Geometry: final body of the model. Coordinates: model frame, mm. A direction names the side the tool comes from. Coordinates: 2 decimals unless noted, no trailing zeros. Loops run counter-clockwise (first coordinate to the right, second up) from the corner with the lowest first, then second, coordinate; pieces in that order, holes last. Notation, with made-up numbers: (-12.5, -22.75) - (29.5, -22.75) arc R28 cw to (29.5, 15.25) - close; hole circle Ø2 at (12.25, 51.25). An arc over 180 degrees is marked (long way). Return JSON: item names as keys, results as strings.
Autodesk Inventor part; units mm, degrees
ref_plane "YZ Plane" through (0, 0, 0) normal (1, 0, 0) x (0, 1, 0)
ref_plane "XZ Plane" through (0, 0, 0) normal (0, 1, 0) x (-1, 0, 0)
ref_plane "XY Plane" through (0, 0, 0) normal (0, 0, 1) x (1, 0, 0)
sketch "Sketch1" plane through (0, 0, 0) normal (0, 0, 1) x (1, 0, 0)
  line L0 (393.6245, -95.4118) -> (-70.3755, -95.4118)
  line L1 (-70.3755, 4.5882) -> (17.6245, 4.5882)
  line L2 (117.6245, 4.5882) -> (205.6245, 4.5882)
  line L3 (305.6245, 4.5882) -> (393.6245, 4.5882)
  line L4 (-88.3755, -15.4118) -> (-70.3755, -15.4118)
  line L5 (-70.3755, -75.4118) -> (-88.3755, -75.4118)
  line L6 (-88.3755, -75.4118) -> (-88.3755, -15.4118)
  line L7 (-70.3755, -95.4118) -> (-70.3755, -75.4118)
  line L8 (-70.3755, -15.4118) -> (-70.3755, 4.5882)
  line L9 (393.6245, -15.4118) -> (411.6245, -15.4118)
  line L10 (411.6245, -15.4118) -> (411.6245, -75.4118)
  line L11 (411.6245, -75.4118) -> (393.6245, -75.4118)
  line L12 (393.6245, 4.5882) -> (393.6245, -15.4118)
  line L13 (393.6245, -75.4118) -> (393.6245, -95.4118)
  line L14 (17.6245, 4.5882) -> (117.6245, 4.5882)
  line L15 (205.6245, 4.5882) -> (305.6245, 4.5882)
  point P0 (0, 0)
  dimension "d0" = 464
  dimension "d4" = 100
  dimension "d9" = 100
  dimension "d13" = 18
  dimension "d14" = 60
  dimension "d17" = 20
  dimension "d19" = 60
  dimension "d20" = 18
  dimension "d21" = 100
extrude "Extrusion1" add sketch "Sketch1" along normal blind 18
sketch "Sketch3" plane through (0, 0, 18) normal (0, 0, 1) x (1, 0, 0)
  line L0 (-70.3755, -15.4118) -> (-71.5069, -14.2805)
  line L1 (-70.3755, -15.4118) -> (-68.7755, -15.4118) construction
  line L2 (-70.3755, -75.4118) -> (-71.5069, -76.5432)
  line L3 (393.6245, -15.4118) -> (394.7558, -14.2805)
  line L4 (393.6245, -75.4118) -> (394.7558, -76.5432)
  circle A0 centre (-71.5069, -14.2805) radius 1.6
  circle A1 centre (-71.5069, -76.5432) radius 1.6
  circle A2 centre (394.7558, -14.2805) radius 1.6
  circle A3 centre (394.7558, -76.5432) radius 1.6
  point P0 (0, 0)
  dimension "d40" = 1.6
  dimension "d41" = 135
  dimension "d42" = 3.2
  dimension "d43" = 3.2
  dimension "d44" = 3.2
  dimension "d45" = 3.2
extrude "Extrusion3" cut sketch "Sketch3" against normal blind 20
properties part number "vigas" material "Wood (Birch)"
Item 1: Section query B-B, the plane y = -5.5. Return loops of the section in (x, z).
Worked out:
{"outline": "(-70.38, 0) - (393.62, 0) - (393.62, 18) - (-70.38, 18) - close"}
Item 2: Ray query, probe 1 along X at (y, z) = (-5.5, 14.75); probe 2 along X at (y, z) = (-15, 11.75). Return the intervals inside material, ascending. Write a range as from..to.
Worked out:
{"probe 1": "-70.38..393.62", "probe 2": "-70.08..393.33"}
Item 3: First-contact query: pin 1 Ø5.5 at (y, z) = (-3, 8) entering from -X; pin 2 Ø8 at (x, z) = (407.5, 7.5) entering from +Y; pin 3 Ø9 at (y, z) = (-86.5, 9) entering from +X. Flat tips, straight axial feed; report the tip coordinate or a pass-through.
Worked out:
{"pin 1": "x = -70.38", "pin 2": "y = -15.41", "pin 3": "x = 393.62"}
Item 4: Section query A-A, the plane z = 9.75. Return loops of the section in (x, y), and give its area (3 significant figures).
Worked out:
{"outline": "(-88.38, -75.41) - (-72.64, -75.41) arc R1.6 cw to (-70.38, -77.67) - (-70.38, -95.41) - (393.62, -95.41) - (393.62, -77.67) arc R1.6 cw to (395.89, -75.41) - (411.62, -75.41) - (411.62, -15.41) - (395.89, -15.41) arc R1.6 cw to (393.62, -13.15) - (393.62, 4.59) - (-70.38, 4.59) - (-70.38, -13.15) arc R1.6 cw to (-72.64, -15.41) - (-88.38, -15.41) - close", "area": "48,600 mm^2"}
Item 5: Reachability of faces 1 (the face through (-81, -15.412, 9)), 2 (the face through (404, -15.412, 9)), 3 (the face through (-70.376, -87, 9)), 4 (the face through (-88.376, -46, 9)), 5 (the face through (404, -75.412, 9)) from +Z, -Z, +X, -X, +Y, -Y: full face, straight path, thin tool, end or side. Return the list, or none.
Worked out:
{"face 1": "+Z, -Z, -X, +Y", "face 2": "+Z, -Z, +X, +Y", "face 3": "+Z, -Z, -X, -Y", "face 4": "+Z, -Z, -X, +Y, -Y", "face 5": "+Z, -Z, +X, -Y"}
